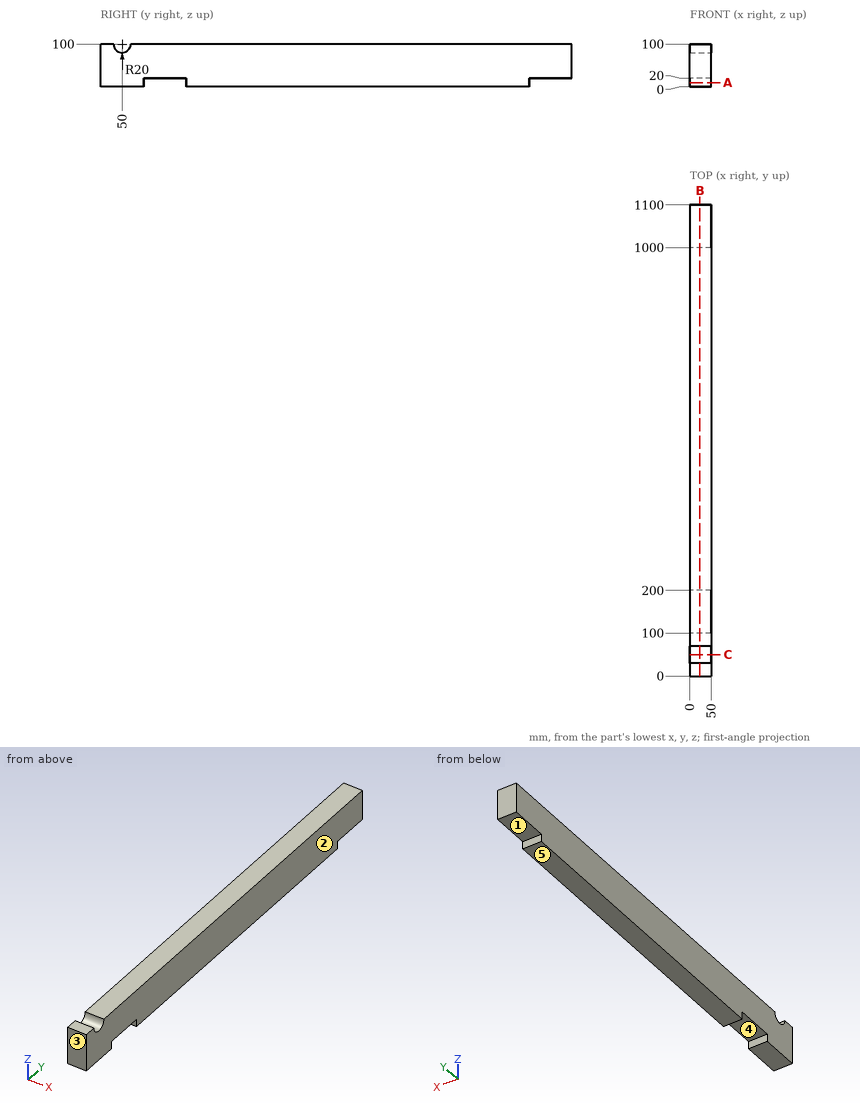
Verification items for this drawing (mm, ordinates from the low corner). A direction names the side the tool comes from. Give positions to 0.01 mm unless a question says otherwise; leave off trailing zeros. Loops run counter-clockwise (first coordinate to the right, second up) from the corner with the lowest first, then second, coordinate; pieces in that order, holes last. Notation, with made-up numbers: M 23.25,-7.75 L 51.25,-7.75 A20 cw 51.25,-1.75 Z; hole C 39,23.5 d6. An arc over 180 degrees is marked long. Answer as a JSON object with one key per item and string values. Group by question number.
Q1. Cross-section at B-B on x = 23.5. Record the cut outline in (y, z).
Q2. Material ranges on line 1 along Y through (x, z) = (46.5, 11); line 2 along Z through (x, y) = (32, 154); line 3 along Y through (x, z) = (5, 89), recorded low to high. Write a range as [from, to].
Q3. Cross-section at C-C on y = 50. Record the cut outline in (x, z).
Q4. Cross-section at A-A on z = 10. Record the cut outline in (x, y).
Q5. Access from +Z, -Z, +X, -X, +Y, -Y to the whole of each face (thin tool, end or side, straight path). Record for the marked faces 1 and 2.
Q6. Release check for a two-part mould opening along Y. For the marked faces 3, 4 and 5 record: released by +Y, released by -Y, zero draft, split by the parting line, or undercut.
Q7. Go/stop test with flat-tipped pins: P1, Ø10, axis at x = 14.5, z = 7, coming from the +Y side; P2, Ø15, axis at x = 23.5, y = 1055, coming from the -Z side. Record where each tip stops, or that it passes through.
Evaluation:
{
 "1": {"outline": "M 0,0 L 100,0 L 100,20 L 200,20 L 200,0 L 1000,0 L 1000,20 L 1100,20 L 1100,100 L 70,100 A20 cw 30,100 L 0,100 Z"},
 "2": {"line 1": "y = [0, 100], [200, 1000]", "line 2": "z = [20, 100]", "line 3": "y = [0, 33.3], [66.7, 1100]"},
 "3": {"outline": "M 0,0 L 50,0 L 50,80 L 0,80 Z"},
 "4": {"outline": "M 0,0 L 50,0 L 50,100 L 0,100 Z; M 0,200 L 50,200 L 50,1000 L 0,1000 Z"},
 "5": {"face 1": "-Z, +X, -X, +Y", "face 2": "+Z, -Z, +X, +Y, -Y"},
 "6": {"face 3": "released by -Y", "face 4": "undercut", "face 5": "zero draft"},
 "7": {"P1": "stops at y = 1000", "P2": "stops at z = 20"}
}
